Build history of the part. All positions in model axes, mm. A direction names the side the tool comes from. Round coordinates to 2 decimals unless told otherwise and drop trailing zeros. Loops run counter-clockwise (first coordinate to the right, second up) from the corner with the lowest first, then second, coordinate; pieces in that order, holes last. Notation, with made-up numbers: M 71,84.5 L 105,84.5 A23 cw 105,107.5 Z; hole C 75.5,-13 d3. An arc over 180 degrees is marked long. Use one line per item in the form item = value. Start each with the question number.
```python
from build123d import *

# Parameters (mm, degrees)
SKETCH1_R           = 37.465
SKETCH1_R_2         = 3.81
BOSS_EXTRUDE1_DEPTH = 2.54
SKETCH2_R           = 9.39
SKETCH2_R_2         = 5.58
BOSS_EXTRUDE2_DEPTH = 50.8
SKETCH3_R           = 37.465
SKETCH3_R_2         = 36.165
BOSS_EXTRUDE3_DEPTH = 49.53
SKETCH5_R           = 5.58
BOSS_EXTRUDE4_DEPTH = 41.91


with BuildPart() as part:
    # Sketch1 → Boss-Extrude1 (new body)
    with BuildSketch(Plane(origin=(0, 0, 0), x_dir=(1, 0, 0), z_dir=(0, 1, 0))):
        with Locations(Location((0, 0, 0), (0, 0, 270))):
            Circle(SKETCH1_R)
        with Locations(Location((0, 0, 0), (0, 0, 270))):
            Circle(SKETCH1_R_2, mode=Mode.SUBTRACT)
    extrude(amount=-BOSS_EXTRUDE1_DEPTH)

    # Sketch2 → Boss-Extrude2 (add)
    # profile 1 of 2: a face of its own
    with BuildSketch(Plane.XZ.offset(2.54)):
        with Locations(Location((0, 18.7325, 0), (0, 0, 90))):
            Circle(SKETCH2_R)
        with Locations(Location((0, 18.7325, 0), (0, 0, 270))):
            Circle(SKETCH2_R_2, mode=Mode.SUBTRACT)
    # profile 2 of 2: a face of its own
    with BuildSketch(Plane.XZ.offset(2.54)):
        with Locations(Location((0, -18.7325, 0), (0, 0, 90))):
            Circle(SKETCH2_R)
        with Locations(Location((0, -18.7325, 0), (0, 0, 90))):
            Circle(SKETCH2_R_2, mode=Mode.SUBTRACT)
    extrude(amount=BOSS_EXTRUDE2_DEPTH)

    # Sketch3 → Boss-Extrude3 (add)
    with BuildSketch(Plane.XZ.offset(2.54)):
        with Locations(Location((0, 0, 0), (0, 0, 90))):
            Circle(SKETCH3_R)
        with Locations(Location((0, 0, 0), (0, 0, 90))):
            Circle(SKETCH3_R_2, mode=Mode.SUBTRACT)
    extrude(amount=BOSS_EXTRUDE3_DEPTH)

    # Sketch5 → Boss-Extrude4 (add)
    with BuildSketch(Plane.XZ.offset(2.54)):
        with Locations(Location((0, 18.7325, 0), (0, 0, 270))):
            Circle(SKETCH5_R)
        with Locations(Location((0, -18.7325, 0), (0, 0, 90))):
            Circle(SKETCH5_R)
    extrude(amount=BOSS_EXTRUDE4_DEPTH)


solid = part.part
```
Q1. Pull direction X, two halves, no side cores. Call faces 3 (the face through (36.574, -25.671, -8.122)), 4 (the face through (0, -44.45, -19)), 5 (the face through (-8, 0, -1)): pulls with the +X half, pulls with the -X half, needs draft (parallel to the pull), parting line crosses it, or undercut.
Q2. Drop flat-ended pins along their axis: P1, Ø12, axis at x = 6.5, y = -24, coming from the +Z side; P2, Ø12, axis at x = -8, z = 27.5, coming from the +Y side; P3, Ø5, axis at x = -16, y = -44, coming from the +Z side; P4, Ø2, axis at x = -8.5, y = -40.5, coming from the -Z side. Give the stop position or say it passes through.
Q3. Tool access for faces 1 (the face through (4, -53.34, 23)), 2 (the face through (-2.821, -27.584, -9.776)): list every direction of +Z, -Z, +X, -X, +Y, -Y with a clear straight run to the whole face (end or side of a thin tool).
Q4. Saw through at D-D (x = 20.5). Give the cut face in (y, z).
Q5. Wall check: probe 1 along X at (y, z) = (-1, 0) (3 decimals); probe 2 along X at (y, z) = (-16, 0) (3 decimals); probe 3 along X at (y, z) = (-23.5, 18.5). Give the ranges that are in metal, low to high.
Q6. Saw through at C-C (z = 0). Give the cut face in (x, y) (3 decimals), and give its area (3 significant figures).
Q7. Saw through at B-B (y = -18.5). Give the cut face in (x, z) (1 decimal).
Filled in:
q1.face_3 = parting line crosses it
q1.face_4 = undercut
q1.face_5 = needs draft
q2.P1 = 37.46
q2.P2 = 0
q2.P3 = 34.95
q2.P4 = -36.71
q3.face_1 = +Z, -Z, +X, -X, -Y
q3.face_2 = -Y
q4.outline = M -52.07,-31.36 L 0,-31.36 L 0,31.36 L -52.07,31.36 L -52.07,29.79 L -2.54,29.79 L -2.54,-29.79 L -52.07,-29.79 Z
q5.probe_1 = -37.465 to -3.81, 3.81 to 37.465
q5.probe_2 = -37.465 to -36.165, 36.165 to 37.465
q5.probe_3 = -32.58 to -31.08, -9.39 to 9.39, 31.08 to 32.58
q6.outline = M -37.465,-52.07 L -36.165,-52.07 L -36.165,-2.54 L -3.81,-2.54 L -3.81,0 L -37.465,0 Z; M 3.81,-2.54 L 36.165,-2.54 L 36.165,-52.07 L 37.465,-52.07 L 37.465,0 L 3.81,0 Z
q6.area = 300 mm²
q7.outline = C 0,0 d74.9; C 0,-18.7 d18.8; C 0,18.7 d18.8; hole C 0,0 d72.3
